Could you check a few things on this model? Use its own coordinates, in mm. Face numbers are marked on the shaded views. A direction names the side the tool comes from. Round coordinates to 2 decimals unless told otherwise and drop trailing zeros. Loops run counter-clockwise (first coordinate to the right, second up) from the corner with the lowest first, then second, coordinate; pieces in that order, holes last. Notation, with made-up numbers: M -34.75,81.25 L 6.25,81.25 A14 ccw 6.25,87.25 Z; hole C -38.75,15 d2. An arc over 180 degrees is marked long. Return JSON: item names as keys, results as strings. Group by question number.
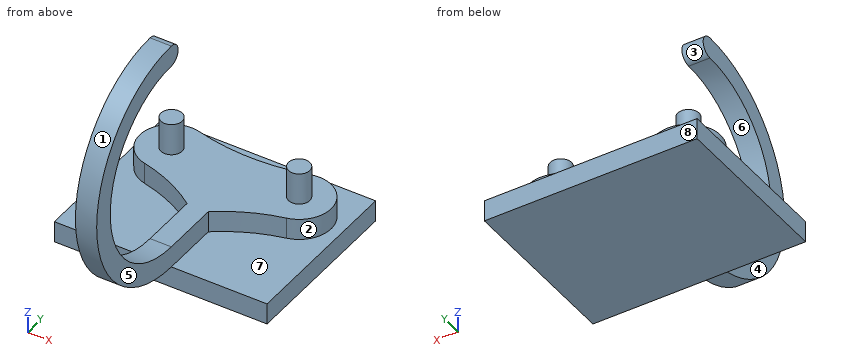
```python
from build123d import *

# Parameters (mm, degrees)
BOSS_EXTRUDE1_DEPTH = 2
SKETCH1_4_R         = 1
BOSS_EXTRUDE2_DEPTH = 4
SKETCH1_6_R         = 1
BOSS_EXTRUDE3_DEPTH = 7
BOSS_EXTRUDE4_DEPTH = 2


with BuildPart() as part:
    # Sketch1 → Boss-Extrude1 (new body)
    with BuildSketch(Plane.XY):
        with BuildLine():
            Line((-10, 8), (-10, -8))
            Line((-10, -8), (-1, -8))
            Line((-1, -8), (-1, -2.549928775))
            ThreePointArc((-1, -2.549928775), (-3.695211651, -0.939284269), (-6.666666667, 0.075011871))
            ThreePointArc((-6.666666667, 0.075011871), (-8.911132412, 3.724781401), (-5.217391304, 5.896122171))
            ThreePointArc((-5.217391304, 5.896122171), (0, 5.203603311), (5.217391304, 5.896122171))
            ThreePointArc((5.217391304, 5.896122171), (8.911132412, 3.724781401), (6.666666667, 0.075011871))
            ThreePointArc((6.666666667, 0.075011871), (3.695211651, -0.939284269), (1, -2.549928775))
            Line((1, -2.549928775), (1, -8))
            Line((1, -8), (10, -8))
            Line((10, -8), (10, 8))
            Line((10, 8), (-10, 8))
        make_face()
    extrude(amount=BOSS_EXTRUDE1_DEPTH)

    # Sketch1<4> → Boss-Extrude2 (add)
    with BuildSketch(Plane.XY):
        with BuildLine():
            Line((-1, -2.549928775), (-1, -8))
            Line((-1, -8), (1, -8))
            Line((1, -8), (1, -2.549928775))
            ThreePointArc((1, -2.549928775), (3.695211651, -0.939284269), (6.666666667, 0.075011871))
            ThreePointArc((6.666666667, 0.075011871), (8.911132412, 3.724781401), (5.217391304, 5.896122171))
            ThreePointArc((5.217391304, 5.896122171), (0, 5.203603311), (-5.217391304, 5.896122171))
            ThreePointArc((-5.217391304, 5.896122171), (-8.911132412, 3.724781401), (-6.666666667, 0.075011871))
            ThreePointArc((-6.666666667, 0.075011871), (-3.695211651, -0.939284269), (-1, -2.549928775))
        make_face()
        with Locations((-6, 3)):
            Circle(SKETCH1_4_R, mode=Mode.SUBTRACT)
        with Locations((6, 3)):
            Circle(SKETCH1_4_R, mode=Mode.SUBTRACT)
    extrude(amount=BOSS_EXTRUDE2_DEPTH)

    # Sketch1<6> → Boss-Extrude3 (add)
    with BuildSketch(Plane.XY):
        with Locations((-6, 3)):
            Circle(SKETCH1_6_R)
        with Locations((6, 3)):
            Circle(SKETCH1_6_R)
    extrude(amount=BOSS_EXTRUDE3_DEPTH)

    # Sketch2 → Boss-Extrude4 (add)
    with BuildSketch(Plane(origin=(1, 0, 0), x_dir=(0, 0, -1), z_dir=(1, 0, 0))):
        with BuildLine():
            Line((-2, -8), (-4, -8))
            ThreePointArc((-4, -8), (-13, -17), (-22, -8))
            ThreePointArc((-22, -8), (-23, -7), (-24, -8))
            ThreePointArc((-24, -8), (-13, -19), (-2, -8))
        make_face()
    extrude(amount=-BOSS_EXTRUDE4_DEPTH)


solid = part.part
```
1. If we section it at D-D, the plane x = -4: Please give me the cut outline in (y, z).
2. If we section it at B-B, the plane y = -12.5: Please give me the cut outline in (x, z).
3. I'm going to push flat-ended pins straight in: pin 1 Ø8 at (x, z) = (6.5, 7) entering from +Y; pin 2 Ø1.6 at (x, y) = (-6, 3.5) entering from +Z; pin 3 Ø3 at (x, y) = (0.5, -6) entering from +Z. Where does each tip first touch, or does it pass through?
4. I need wall thicknesses on probe 1 along Z at (x, y) = (-1.5, 1.75); probe 2 along X at (y, z) = (-9.25, 4); probe 3 along Z at (x, y) = (-4, -5.5). Which ranges of each line are inside material? Lowest first, please.
5. On a 3-axis mill with a long thin cutter (end or side, diameter ignored), from which of +Z, -Z, +X, -X, +Y, -Y can I reach the whole of each face in a straight line? I mean the marked faces 4, 5, 6, 7 and 8. Say none if no direction works.
6. If we section it at A-A, the plane y = -6.5: Please give me the cut outline in (x, z).
7. We'd pull the mould along Z, two halves only. Please class the marked faces 1, 2 and 3: +Z half, -Z half, draft (parallel to the pull), parting line (faces both ways), or undercut.
8. If we section it at C-C, the plane z = 5.5: Please give me the cut outline in (x, y).
Geometry results:
{
 "1": {"outline": "M -8,0 L 8,0 L 8,2 L 5.61,2 L 5.61,4 L -0.8,4 L -0.8,2 L -8,2 Z"},
 "2": {"outline": "M -1,2.96 L 1,2.96 L 1,5.21 L -1,5.21 Z; M -1,20.79 L 1,20.79 L 1,23.04 L -1,23.04 Z"},
 "3": {"pin 1": "y = 6", "pin 2": "z = 7", "pin 3": "z = 23.87"},
 "4": {"probe 1": "0 to 4", "probe 2": "-1 to 1", "probe 3": "0 to 2"},
 "5": {"face 4": "+Z, -X, -Y", "face 5": "+Z, +X, -Y", "face 6": "+X, -X, +Y", "face 7": "+Z", "face 8": "+Z, -Z, +X, -X, +Y"},
 "6": {"outline": "M -10,0 L 10,0 L 10,2 L 1,2 L 1,4 L -1,4 L -1,2 L -10,2 Z"},
 "7": {"face 1": "parting line", "face 2": "draft", "face 3": "undercut"},
 "8": {"outline": "C -6,3 d2; M -1,-16.05 L 1,-16.05 L 1,-12.97 L -1,-12.97 Z; C 6,3 d2"}
}
